```python
from build123d import *

# Parameters (mm, degrees)
F2_R = 2.54


with BuildPart() as f1:
    # F0 (on Front) → F1 (revolve)
    with BuildSketch(Plane.XZ):
        with BuildLine():
            Line((50.4768975079, 61.4194460213), (0, 0))
            Line((0, 0), (0, -63.5373517871))
            Line((0, -63.5373517871), (15.5935517171, -63.5373517871))
            Line((15.5935517171, -63.5373517871), (15.5935517171, -16.9645253417))
            ThreePointArc((15.5935517171, -16.9645253417), (18.9662168832, -2.8402970726), (28.3564869314, 8.2363234833))
            Line((28.3564869314, 8.2363234833), (50.4768975079, 24.4736485183))
            Line((50.4768975079, 24.4736485183), (50.4768975079, 61.4194460213))
        make_face()
    revolve(axis=Axis((0, 0, 22.0490116626), (0, 0, 1)))

    # F2
    f2_edges = [f1.edges().sort_by_distance(p)[0] for p in [
        (-50.476898, 0, 61.419446),
        (-50.476898, 0, 24.473649),
    ]]
    fillet(f2_edges, radius=F2_R)


solid = f1.part
```
Here's how the part is built. I have some questions about the finished solid (model axes, mm). Coordinates: 2 decimals unless noted, no trailing zeros. Loops run counter-clockwise (first coordinate to the right, second up) from the corner with the lowest first, then second, coordinate; pieces in that order, holes last. Notation, with made-up numbers: (-36, -35) - (1, -35) arc R33 ccw to (1, -7) - close; hole circle Ø8 at (-25, 6.5). An arc over 180 degrees is marked (long way). Return JSON: item names as keys, results as strings. Group by question number.
Item 1: If we section it at C-C on z = 18.5: Write out the boundary of the cut face in (x, y), and give its area (3 significant figures).
Item 2: I need wall thicknesses on line 1 (Y direction, x = -24, z = 48); line 2 (X direction, y = -5.5, z = -14); line 3 (Z direction, x = -19, y = -9). Which ranges of each line are inside material? Lowest first, please. Write a range as from..to.
Item 3: If we section it at A-A on z = -32: Write out the boundary of the cut face in (x, y).
Item 4: Will these pins go through, and if not, where does the flat tip stop? P1, Ø10, axis at y = -7.5, z = 21, coming from the +X side; P2, Ø4, axis at x = -32, y = 22, coming from the -Z side; P3, Ø8, axis at x = -5.5, z = -24.5, coming from the -Y side; P4, Ø1.5, axis at y = -26, z = 4.5, coming from the +X side.
Item 5: We'd pull the mould along Y, two halves only. Please class faces 1 (the face through (-15.58, 0.69, -39.92)), 2 (the face through (0, 0, -63.537)), 3 (the face through (11.874, 3.739, 15.148)): +Y half, -Y half, draft (parallel to the pull), parting line (faces both ways), or undercut.
Item 6: If we section it at B-B on z = 42: Write out the boundary of the cut face in (x, y).
Calculated:
{
 "1": {"outline": "circle Ø84.68 at (0, 0); hole circle Ø30.41 at (0, 0)", "area": "4,910 mm^2"},
 "2": {"line 1": "y = -44.41..-31.31, 31.31..44.41", "line 2": "x = -14.74..14.74", "line 3": "z = 0.64..25.58"},
 "3": {"outline": "circle Ø31.19 at (0, 0)"},
 "4": {"P1": "stops at x = 50.19", "P2": "stops at z = 14.46", "P3": "stops at y = -15.52", "P4": "passes through"},
 "5": {"face 1": "parting line", "face 2": "draft", "face 3": "undercut"},
 "6": {"outline": "circle Ø100.95 at (0, 0); hole circle Ø69.03 at (0, 0)"}
}
